from build123d import *

# Parameters (mm, degrees)
SKETCH1_R                 = 34.29
BOSS_EXTRUDE1_DEPTH       = 1.6383
SKETCH3_W                 = 3.048
SKETCH3_H                 = 3.048
BOSS_EXTRUDE3_DEPTH       = 4.0767
CIRPATTERN1_COUNT         = 30
F_6_CLEARANCE_HOLE1_D     = 3.7973
F_6_CLEARANCE_HOLE1_DEPTH = 1.6383


with BuildPart() as part:
    # Sketch1 → Boss-Extrude1 (new body)
    with BuildSketch(Plane(origin=(0, 0, 0), x_dir=(1, 0, 0), z_dir=(0, 1, 0))):
        Circle(SKETCH1_R)
    extrude(amount=BOSS_EXTRUDE1_DEPTH)

    # Sketch3 → Boss-Extrude3 (add)
    with BuildSketch(Plane(origin=(0, 1.6383, 0), x_dir=(1, 0, 0), z_dir=(0, 1, 0))):
        with Locations((0, 31.97225)):
            Rectangle(SKETCH3_W, SKETCH3_H)
    boss_extrude3 = extrude(amount=BOSS_EXTRUDE3_DEPTH)

    # CirPattern1: Boss-Extrude3 ×30 about axis
    cirpattern1_axis = Axis((0, 0, 0.08061427), (0, 1, 0))
    for i in range(1, CIRPATTERN1_COUNT):
        add(boss_extrude3.rotate(cirpattern1_axis, i * 360 / CIRPATTERN1_COUNT))

    # #6 Clearance Hole1
    with Locations(Plane(origin=(0, 0, 0), x_dir=(-1, 0, 0), z_dir=(0, -1, 0))):
        with Locations((13.97, -8.89), (13.97, 8.89), (-13.97, 8.89), (-13.97, -8.89)):
            Hole(F_6_CLEARANCE_HOLE1_D / 2, depth=F_6_CLEARANCE_HOLE1_DEPTH)


solid = part.part
Geometry check sheet. Reference: the model listing, model coordinates, mm. A direction names the side the tool comes from. Give positions to 0.01 mm unless a question says otherwise; leave off trailing zeros. Loops run counter-clockwise (first coordinate to the right, second up) from the corner with the lowest first, then second, coordinate; pieces in that order, holes last.
(1) Section check D-D on z = 0. Record the cut outline in (x, y).
From the geometry:
outline: (-34.29, 0) - (34.29, 0) - (34.29, 1.64) - (-34.29, 1.64) - close
(2) Section check B-B on x = 0. Record the cut outline in (y, z) (3 decimals).
From the geometry:
outline: (0, -34.29) - (1.638, -34.29) - (1.638, -33.496) - (5.715, -33.496) - (5.715, -30.448) - (1.638, -30.448) - (1.638, 30.609) - (5.715, 30.609) - (5.715, 33.657) - (1.638, 33.657) - (1.638, 34.29) - (0, 34.29) - close
(3) Release check for a two-part mould opening along X. For faces 4 (the flat face through (30, 5.715, -10)), 5 (the flat face through (31.697, 3.648, 4.944)), 6 (the flat face through (24.97, 3.65, 22.53)) record: released by +X, released by -X, zero draft, split by the parting line, or undercut.
From the geometry:
face 4: zero draft
face 5: undercut
face 6: released by +X
(4) Depth check by flat-ended pin: pin 1 Ø0.9 at (x, y) = (0.5, 4) entering from -Z; pin 2 Ø1 at (x, z) = (-14.5, -7.5) entering from +Y; pin 3 Ø2.5 at (y, z) = (4.5, 32.5) entering from +X. Enter the tip coordinate at first touch or a pass-through.
From the geometry:
pin 1: stops at z = -33.5
pin 2: stops at y = 1.64
pin 3: stops at x = 12.54
(5) Thickness scan on L1, parallel to Z at x = 13.97, y = 0.5; L2, parallel to X at y = 0.4, z = -8.89; L3, parallel to Y at x = -18, z = -12. Record the ranges inside material, lowest first.
From the geometry:
L1: z = -31.32 to -10.79, -6.99 to 6.99, 10.79 to 31.32
L2: x = -33.12 to -15.87, -12.07 to 12.07, 15.87 to 33.12
L3: y = 0 to 1.64
(6) Section check C-C on y = 3.85. Count the separate pieces of the cut face and the enclosed holes in it, then the cut area to 3 significant figures.
From the geometry:
separate pieces: 30
enclosed holes: 0
area: 279 mm2
(7) Section check A-A on z = -10. Record the cut outline in (x, y) (3 decimals), then the cut area to 3 significant figures.
From the geometry:
outline: (-32.799, 0) - (-15.51, 0) - (-15.51, 1.638) - (-28.825, 1.638) - (-28.825, 5.715) - (-32.029, 5.715) - (-32.029, 1.638) - (-32.799, 1.638) - close; (-12.43, 0) - (12.43, 0) - (12.43, 1.638) - (-12.43, 1.638) - close; (15.51, 0) - (32.799, 0) - (32.799, 1.638) - (32.029, 1.638) - (32.029, 5.715) - (28.825, 5.715) - (28.825, 1.638) - (15.51, 1.638) - close
area: 124 mm2
(8) Set-up check for faces 1 (the flat face through (24.8, 3.6, -20.2)), 2 (the flat face through (19.8, 3.6, 27.2)), 3 (the flat face through (-6.368, 3.648, -29.777)): record each of +Z, -Z, +X, -X, +Y, -Y from which the full face is reachable in a straight line by a thin tool's end or side.
From the geometry:
face 1: +X, +Y
face 2: +Z, +X, +Y
face 3: +Y
